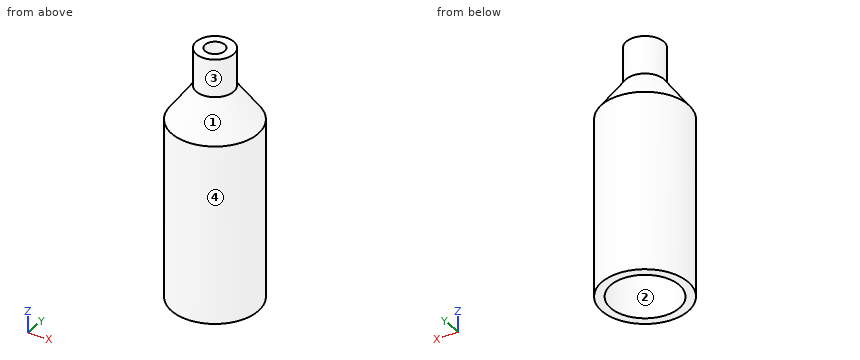
Solid Edge part; units mm, degrees
sketch "Sketch1" plane through (0, 0, 0) normal (0, 0, 1) x (1, 0, 0)
  circle A0 centre (0, 0) radius 3.85
  circle A1 centre (0, 0) radius 4.85
extrude "ProtrusiónExtruida_22" add sketch "Sketch1" along normal blind 20
sketch "Sketch2" plane through (0, 0, 0) normal (0, -1, 0) x (1, 0, 0)
  line L0 (1.1, 28.0416) -> (1.1, 23.893)
  line L1 (1.1, 23.893) -> (3.9054, 20)
  line L2 (4.85, 20) -> (3.9054, 20)
  line L3 (4.85, 20) -> (2.1, 23.8161)
  line L4 (2.1, 28.0416) -> (2.1, 23.8161)
  line L5 (1.1, 28.0416) -> (2.1, 28.0416)
revolve "RevolvedProtrusion1" add sketch "Sketch2" angle 360 about axis through (0, 0, 54) along (0, 0, -1)
Input: part model. Units: mm. Frame: model coordinates. Face numbers are marked on the shaded views. A direction names the side the tool comes from. Round coordinates to 2 decimals unless told otherwise and drop trailing zeros. Loops run counter-clockwise (first coordinate to the right, second up) from the corner with the lowest first, then second, coordinate; pieces in that order, holes last. Notation, with made-up numbers: (77, -17.75) -> (85, -17.75) arc R17 cw to (85, -6.75) -> close; hole circle Ø8 at (-15, 63). An arc over 180 degrees is marked (long way). Answer as a JSON object with one key per item and string values. Group by question number.
1) Reachability of the marked faces 3 and 4 from +Z, -Z, +X, -X, +Y, -Y: full face, straight path, thin tool, end or side. Return the list, or none.
2) Draft query along X for the marked faces 1 and 2. Return one class per face: +X half, -X half, draft (parallel to the pull), parting line (faces both ways), or undercut.
3) Section query A-A on x = 0. Output: boundary loops of the cut face in (y, z), plus the area to 3 significant figures.
4) Section query D-D on z = 21. Output: boundary loops of the cut face in (x, y), plus the area to 3 significant figures.
5) Pin query (flat end, axial travel): pin 1 (1.8 mm diameter, centred on x = 0, y = 0, fed in from +Z); pin 2 (5 mm diameter, centred on x = 0.5, y = -1, fed in from -Z); pin 3 (4.5 mm diameter, centred on x = 0, y = 0, fed in from -Z); pin 4 (1 mm diameter, centred on x = -1.5, z = 16, fed in from +Y). Return the tip coordinate at first contact, or that it passes through.
6) Ray query, L1, parallel to X at y = 0, z = 25.1; L2, parallel to Y at x = 0, z = 15. Return the intervals inside material, ascending.
7) Section query C-C on z = 8.75. Output: boundary loops of the cut face in (x, y), plus the area to 3 significant figures.
Reply:
{
 "1": {"face 3": "+Z", "face 4": "+Z, -Z"},
 "2": {"face 1": "parting line", "face 2": "undercut"},
 "3": {"outline": "(-4.85, 0) -> (-3.85, 0) -> (-3.85, 20) -> (-3.91, 20) -> (-1.1, 23.89) -> (-1.1, 28.04) -> (-2.1, 28.04) -> (-2.1, 23.82) -> (-4.85, 20) -> close; (1.1, 23.89) -> (3.91, 20) -> (3.85, 20) -> (3.85, 0) -> (4.85, 0) -> (4.85, 20) -> (2.1, 23.82) -> (2.1, 28.04) -> (1.1, 28.04) -> close", "area": "55.7 mm2"},
 "4": {"outline": "circle Ø8.26 at (0, 0); hole circle Ø6.37 at (0, 0)", "area": "21.7 mm2"},
 "5": {"pin 1": "passes through", "pin 2": "stops at z = 20.4", "pin 3": "stops at z = 22.3", "pin 4": "stops at y = 4.75"},
 "6": {"L1": "x = -2.1 to -1.1, 1.1 to 2.1", "L2": "y = -4.85 to -3.85, 3.85 to 4.85"},
 "7": {"outline": "circle Ø9.7 at (0, 0); hole circle Ø7.7 at (0, 0)", "area": "27.3 mm2"}
}
